Solid Edge part; units mm, degrees
sketch "Sketch1" plane through (0, 0, 0) normal (0, 0, 1) x (1, 0, 0)
  line L0 (-2.8868, -5) -> (2.8868, -5)
  line L1 (2.8868, -5) -> (5.7735, 0)
  line L2 (5.7735, 0) -> (2.8868, 5)
  line L3 (2.8868, 5) -> (-2.8868, 5)
  line L4 (-2.8868, 5) -> (-5.7735, 0)
  line L5 (-5.7735, 0) -> (-2.8868, -5)
extrude "Protrusion1" add sketch "Sketch1" along normal blind 5.1
sketch "Sketch2" plane through (0, 0, 0) normal (0, -1, 0) x (1, 0, 0)
  line L0 (-5, 5.1) -> (-5.7735, 4.6534)
revolve "RevolvedCutout1" cut sketch "Sketch2" angle 360 about axis through (0, 0, 57.15) along (0, 0, -1) material side at (-5.4118, 0, 4.92)
sketch "Sketch3" plane through (0, 0, 0) normal (0, -1, 0) x (1, 0, 0)
  line L0 (-5, 0) -> (-5.7735, 0.4466)
revolve "RevolvedCutout2" cut sketch "Sketch3" angle 360 about axis through (0, 0, 57.15) along (0, 0, -1) material side at (-5.4118, 0, 0.18)
sketch "Sketch4" plane through (0, 0, 0) normal (0, 0, 1) x (1, 0, 0)
  circle A0 centre (0, 0) radius 2.4585
extrude "Cutout1" cut sketch "Sketch4" along normal through all and the other way through all
chamfer "Chamfer1" distance 0.5 angle 45 2 edges at (-2.4585, 0, 5.1) (-2.4585, 0, 0)
cosmetic_thread "Thread1"
properties material "Steel"
The model under review builds one solid part; all positions refer to its coordinate system, in mm. Coordinates: 2 decimals unless noted, no trailing zeros. Loops run counter-clockwise (first coordinate to the right, second up) from the corner with the lowest first, then second, coordinate; pieces in that order, holes last. Notation, with made-up numbers: (9, 74.5) -> (28, 74.5) arc R21 cw to (28, 103.5) -> close; hole circle Ø9 at (82, -14.75). An arc over 180 degrees is marked (long way). Use a Markdown table: item, result. Add a question column.
1. Draft analysis for pull direction X (two halves, no side actions). For faces 1 (the face through (2.2, -2.2, 0)), 2 (the face through (-4.35, -2.465, 2.514)), 3 (the face through (2.345, -0.738, 2.521)), state which applies: pulls with the +X half, pulls with the -X half, needs draft (parallel to the pull), parting line crosses it, or undercut.
2. To check wall thickness, follow line 1 (Y direction, x = 0, z = 2.2); line 2 (X direction, y = 1.25, z = 2.25); line 3 (Y direction, x = -1.25, z = 1.6). State the ranges of each line that lie inside material, in increasing order.
3. Add section A-A on z = 2.1. Write out the cut boundary in (x, y).
4. Clearance check with flat-ended pins moving along their axes: pin 1 Ø1 at (y, z) = (-2.5, 4.5) entering from +X; pin 2 Ø1.5 at (y, z) = (-1, 3) entering from -X; pin 3 Ø4.5 at (x, y) = (0, 0) entering from -Z. State where each tip first meets the part, or that it passes through.
Returned:
| question | item | result |
|---|---|---|
| 1 | face 1 | needs draft |
| 1 | face 2 | pulls with the -X half |
| 1 | face 3 | undercut |
| 2 | line 1 | y = -5 to -2.46, 2.46 to 5 |
| 2 | line 2 | x = -5.05 to -2.12, 2.12 to 5.05 |
| 2 | line 3 | y = -5 to -2.12, 2.12 to 5 |
| 3 | outline | (-5.77, 0) -> (-2.89, -5) -> (2.89, -5) -> (5.77, 0) -> (2.89, 5) -> (-2.89, 5) -> close; hole circle Ø4.92 at (0, 0) |
| 4 | pin 1 | stops at x = 4.62 |
| 4 | pin 2 | stops at x = -5.63 |
| 4 | pin 3 | passes through |
